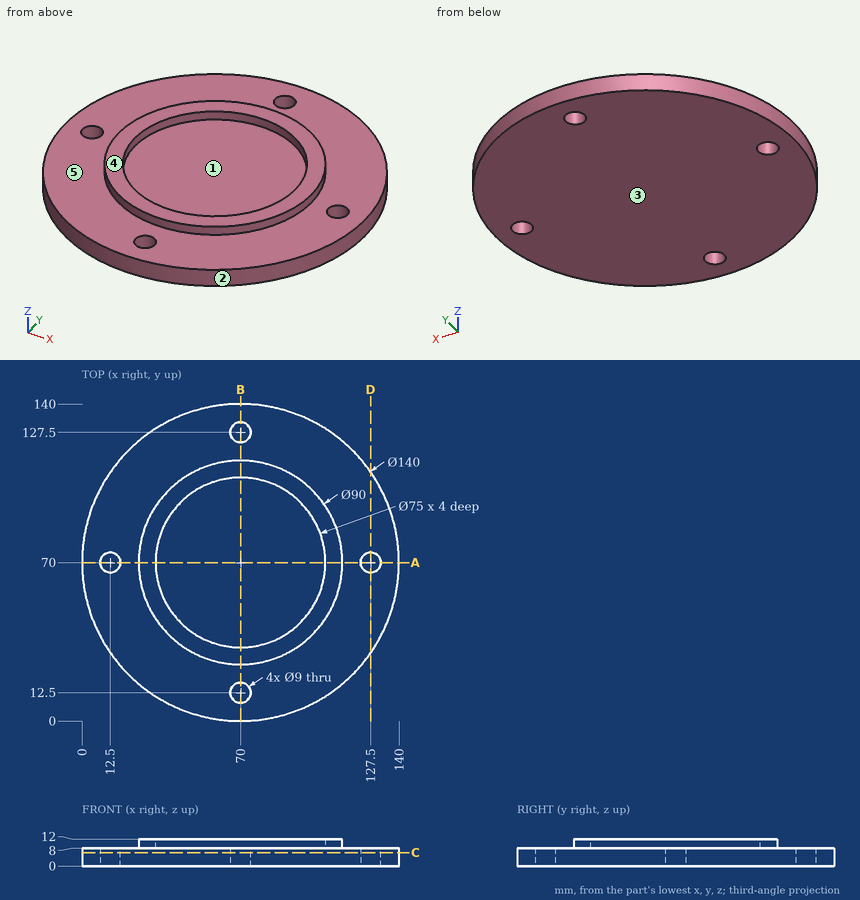
Study the drawing (mm; zero at the part's minimum x, y, z) and answer. A direction names the side the tool comes from. Coordinates: 2 decimals unless noted, no trailing zeros. Write each loop counter-clockwise with the first axis right and the second up, starting at its lowest first coordinate (ties: lowest second). Pieces come first, ordered by that corner, then holes. Notation, with made-up numbers: (-40, 28.5) - (-9, 28.5) arc R27 ccw to (-9, 53.5) - close; hole circle Ø10 at (-14, 68.25). An arc over 180 degrees is marked (long way). Answer as a JSON object with one key per item and string values.
Q1. Find section D-D (x = 127.5). Write down the section's boundary in (y, z), plus the area to 3 significant figures.
Results list:
{"outline": "(30.08, 0) - (65.5, 0) - (65.5, 8) - (30.08, 8) - close; (74.5, 0) - (109.92, 0) - (109.92, 8) - (74.5, 8) - close", "area": "567 mm^2"}
Q2. Find section A-A (y = 70). Write down the section's boundary in (x, z).
Results list:
{"outline": "(0, 0) - (8, 0) - (8, 8) - (0, 8) - close; (17, 0) - (123, 0) - (123, 8) - (115, 8) - (115, 12) - (107.5, 12) - (107.5, 8) - (32.5, 8) - (32.5, 12) - (25, 12) - (25, 8) - (17, 8) - close; (132, 0) - (140, 0) - (140, 8) - (132, 8) - close"}
Q3. Which of the six approach directions +Z, -Z, +X, -X, +Y, -Y give full straight-line access (tool end or side, diameter ignored) to the marked faces 4 and 5?
Results list:
{"face 4": "+Z, +X, -X, +Y, -Y", "face 5": "+Z"}
Q4. For a pull along X with two mould halves and no side action, classify the marked faces 1, 2 and 3 as pulls with the +X half, pulls with the -X half, needs draft (parallel to the pull), parting line crosses it, or undercut.
Results list:
{"face 1": "undercut", "face 2": "parting line crosses it", "face 3": "needs draft"}
Q5. Consider L1, parallel to Y at x = 70, z = 10.8; L2, parallel to Y at x = 70, z = 5; L3, parallel to Y at x = 71.5, z = 3.5. Determine where each line is inside the solid, lowest interval first. Write a range as from..to.
Results list:
{"L1": "y = 25..32.5, 107.5..115", "L2": "y = 0..8, 17..123, 132..140", "L3": "y = 0.02..8.26, 16.74..123.26, 131.74..139.98"}
Q6. Given pin 1 Ø12 at (x, y) = (111, 26) entering from +Z; pin 2 Ø4 at (x, z) = (61.5, 8.5) entering from -Y, each flat-ended and moving along its own axis, determine where each tip first touches the part or whether it passes through.
Results list:
{"pin 1": "stops at z = 8", "pin 2": "stops at y = 0.31"}
Q7. Find section C-C (z = 6). Write down the section's boundary in (x, y), plus the area to 3 significant figures.
Results list:
{"outline": "circle Ø140 at (70, 70); hole circle Ø9 at (12.5, 70); hole circle Ø9 at (70, 12.5); hole circle Ø9 at (70, 127.5); hole circle Ø9 at (127.5, 70)", "area": "15,100 mm^2"}
